Input: part model. Units: mm. Frame: model coordinates. Coordinates: 2 decimals unless noted, no trailing zeros. Loops run counter-clockwise (first coordinate to the right, second up) from the corner with the lowest first, then second, coordinate; pieces in that order, holes last. Notation, with made-up numbers: M -1.75,-17 L 31.25,-17 A10 cw 31.25,-11 Z; hole C 81,-3 d8. An arc over 180 degrees is marked long. Use a Markdown table: item, result. Add a question column.
1. Line query: L1, parallel to Z at x = -80, y = 1.1; L2, parallel to X at y = 1.35, z = -18.5; L3, parallel to X at y = 1.2, z = -26.6. Output: solid intervals per line, ascending. Write a range as [from, to].
2. Pin query (flat end, axial travel): pin 1 (5.5 mm diameter, centred on x = -80, z = -26.6, fed in from -Y); pin 2 (0.6 mm diameter, centred on y = 1, z = -29, fed in from -X) (3 decimals); pin 3 (0.6 mm diameter, centred on x = 51, y = 1, fed in from -Z). Return the tip coordinate at first contact, or that it passes through.
3. Draft query along X for faces 1 (the flat face through (-1, 0, -3)), 2 (the cylindrical face through (-81.31, 1.01, -25.6)), 3 (the flat face through (-83.48, 0.99, -27.85)), 4 (the cylindrical face through (35.824, 1.014, 23.232)). Return one class per face: +X half, -X half, draft (parallel to the pull), parting line (faces both ways), or undercut.
4. Section D-D on x = -80. Output: boundary loops of the cut face in (y, z).
5. Section A-A on z = -21.5. Output: boundary loops of the cut face in (x, y), then the cut area to 3 significant figures.
6. Section C-C on y = 1.6. State how many separate pieces and enclosed holes the cut face has, then the cut area to 3 significant figures.
7. Section B-B on x = -34.3. Output: boundary loops of the cut face in (y, z), then the cut area to 3 significant figures.
```python
from build123d import *

# Parameters (mm, degrees)
BOSS_EXTRU_1_DEPTH           = 2
ESQUISSE2_R                  = 1.65
ENL_V_MAT_EXTRU_1_DEPTH      = 1
ENL_V_MAT_EXTRU_1_DEPTH_BACK = 3


with BuildPart() as part:
    # Esquisse1 → Boss.-Extru.1 (new body)
    with BuildSketch(Plane(origin=(0, 0, 0), x_dir=(1, 0, 0), z_dir=(0, 1, 0))):
        Polygon((21.9, 26.4), (-21.9, 26.4), (-21.9, 18.1), (-30.5, 18.1), (-30.5, 26.4), (-75.6, 26.4), (-75.6, 31.4), (-82, 31.4), (-85, 24.2), (-85, -26.4), (-30.5, -26.4), (-30.5, -18.1), (-21.9, -18.1), (-21.9, -26.4), (21.9, -26.4), (21.9, -18.1), (30.5, -18.1), (30.5, -26.4), (85, -26.4), (85, 24.2), (82, 31.4), (75.6, 31.4), (75.6, 26.4), (30.5, 26.4), (30.5, 18.1), (21.9, 18.1), align=None)
    extrude(amount=BOSS_EXTRU_1_DEPTH)

    # Esquisse2 → Enlèv. mat.-Extru.1 (cut, two sides)
    with BuildSketch(Plane(origin=(0, 2, 0), x_dir=(1, 0, 0), z_dir=(0, 1, 0))) as enl_v_mat_extru_1_sk:
        with Locations((-80, 26.6)):
            Circle(ESQUISSE2_R)
        with Locations((-34.3, -22.6)):
            Circle(ESQUISSE2_R)
        with Locations((34.3, -22.6)):
            Circle(ESQUISSE2_R)
        with Locations((80, 26.6)):
            Circle(ESQUISSE2_R)
    extrude(amount=ENL_V_MAT_EXTRU_1_DEPTH, mode=Mode.SUBTRACT)
    extrude(enl_v_mat_extru_1_sk.sketch, amount=-ENL_V_MAT_EXTRU_1_DEPTH_BACK, mode=Mode.SUBTRACT)


solid = part.part
```
Answers below:
| question | item | result |
|---|---|---|
| 1 | L1 | z = [-31.4, -28.25], [-24.95, 26.4] |
| 1 | L2 | x = [-85, -30.5], [-21.9, 21.9], [30.5, 85] |
| 1 | L3 | x = [-84, -81.65], [-78.35, -75.6], [75.6, 78.35], [81.65, 84] |
| 2 | pin 1 | stops at y = 0 |
| 2 | pin 2 | stops at x = -83.125 |
| 2 | pin 3 | stops at z = -26.4 |
| 3 | face 1 | draft |
| 3 | face 2 | undercut |
| 3 | face 3 | -X half |
| 3 | face 4 | undercut |
| 4 | outline | M 0,-31.4 L 2,-31.4 L 2,-28.25 L 0,-28.25 Z; M 0,-24.95 L 2,-24.95 L 2,26.4 L 0,26.4 Z |
| 5 | outline | M -85,0 L -30.5,0 L -30.5,2 L -85,2 Z; M -21.9,0 L 21.9,0 L 21.9,2 L -21.9,2 Z; M 30.5,0 L 85,0 L 85,2 L 30.5,2 Z |
| 5 | area | 306 mm² |
| 6 | separate pieces | 1 |
| 6 | enclosed holes | 4 |
| 6 | area | 8,730 mm² |
| 7 | outline | M 0,-26.4 L 2,-26.4 L 2,20.95 L 0,20.95 Z; M 0,24.25 L 2,24.25 L 2,26.4 L 0,26.4 Z |
| 7 | area | 99.0 mm² |
